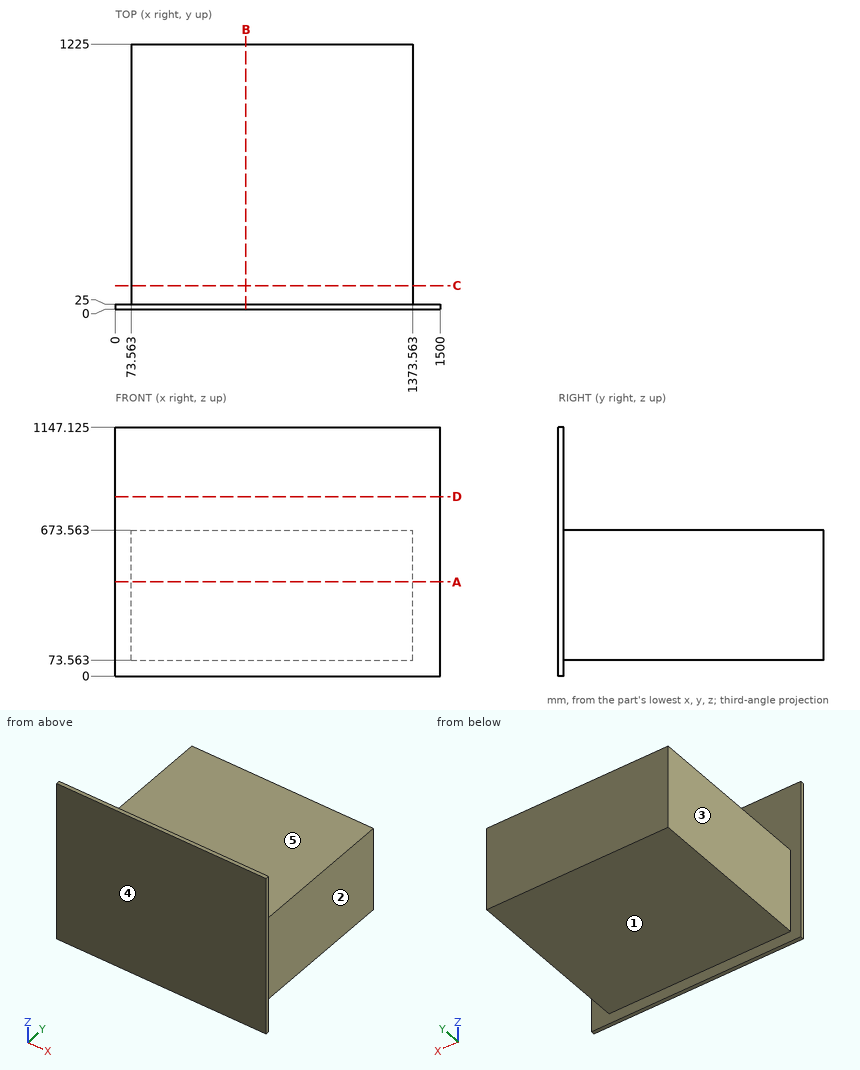
Input: dimensioned drawing with shaded views. Units: mm. Origin: part minimum x, y, z. A direction names the side the tool comes from. Give positions to 0.01 mm unless a question says otherwise; leave off trailing zeros. Write each loop counter-clockwise with the first axis right and the second up, starting at its lowest first coordinate (ties: lowest second). Pieces come first, ordered by that corner, then holes.
1. Access query for the marked faces 1, 2, 3, 4 and 5. Directions: +Z, -Z, +X, -X, +Y, -Y. A direction counts if a zero-diameter tool reaches every point of the face in a straight line with its end or side. Return the directions, or none.
2. Section query C-C (y = 110). Return the cut outline in (x, z).
3. Section query B-B (x = 603). Return the cut outline in (y, z) (1 decimal), then the cut area to 3 significant figures.
4. Section query D-D (z = 828). Return the cut outline in (x, y).
5. Material intervals for line 1 along Y through (x, z) = (827, 1096); line 2 along Z through (x, y) = (1089.5, 655.5); line 3 along X through (y, z) = (333.5, 642), sorted ascending.
6. First-contact query: pin 1 (8 mm diameter, centred on x = 1110.5, y = 903, fed in from -Z); pin 2 (1 mm diameter, centred on x = 451.5, z = 908.5, fed in from -Y). Flat tips, straight axial feed; report the tip coordinate or a pass-through.
7. Section query A-A (z = 434). Return the cut outline in (x, y).
Output values:
1. face 1: -Z, +X, -X, +Y
1. face 2: +Z, -Z, +X, +Y
1. face 3: +Z, -Z, -X, +Y
1. face 4: +Z, -Z, +X, -X, -Y
1. face 5: +Z, +X, -X, +Y
2. outline: (73.56, 73.56) - (1373.56, 73.56) - (1373.56, 673.56) - (73.56, 673.56) - close
3. outline: (0, 0) - (25, 0) - (25, 73.6) - (1225, 73.6) - (1225, 673.6) - (25, 673.6) - (25, 1147.1) - (0, 1147.1) - close
3. area: 749,000 mm2
4. outline: (0, 0) - (1500, 0) - (1500, 25) - (0, 25) - close
5. line 1: y = 0 to 25
5. line 2: z = 73.56 to 673.56
5. line 3: x = 73.56 to 1373.56
6. pin 1: stops at z = 73.56
6. pin 2: stops at y = 0
7. outline: (0, 0) - (1500, 0) - (1500, 25) - (1373.56, 25) - (1373.56, 1225) - (73.56, 1225) - (73.56, 25) - (0, 25) - close
